Verification items for the finished model (mm, model axes). Face numbers are marked on the shaded views. A direction names the side the tool comes from. Coordinates: 2 decimals unless noted, no trailing zeros. Order: outer loops, then holes, each group sorted by start corner. A loop starts at its lowest first (then second) coordinate and runs counter-clockwise, first axis right, second up.
Q1. Cross-section at A-A, the plane z = 0. Record the boundary of the cut face in (x, y) (3 decimals), and give its area (3 significant figures).
Q2. Cross-section at D-D, the plane x = 0. Count the separate pieces of the cut face and the enclosed holes in it, and give its area (3 significant figures).
Q3. Cross-section at B-B, the plane y = 28.5. Record the boundary of the cut face in (x, z), and give its area (3 significant figures).
Q4. Set-up check for the marked faces 5, 6, 7, 8 and 9: record each of +Z, -Z, +X, -X, +Y, -Y from which the full face is reachable in a straight line by a thin tool's end or side.
Q5. Draft check along X on the marked faces 1, 2, 3 and 4. Enter one of: pulls with the +X half, pulls with the -X half, needs draft (parallel to the pull), parting line crosses it, or undercut.
Q6. Cross-section at C-C, the plane x = 34. Record the boundary of the cut face in (y, z) (3 decimals).
Q7. Depth check by flat-ended pin: P1, Ø5, axis at x = -36.5, y = 15.5, coming from the +Z side; P2, Ø12, axis at y = 26.5, z = -25.5, coming from the -X side; P3, Ø1, axis at x = -39, y = -20.5, coming from the +Z side. Enter the tip coordinate at first touch or a pass-through.
Q8. Thickness scan on line 1 (Z direction, x = 0, y = -4.8) (3 decimals); line 2 (Z direction, x = 0, y = 8); line 3 (Z direction, x = 0, y = 17.5). Record the ranges inside material, lowest first.
from build123d import *

# Parameters (mm, degrees)
F0_R      = 52.07
F1_DEPTH  = 5.08
F0_R_2    = 55.245
F2_DEPTH  = 30.48
F4_DEPTH  = 21.59
F5_W      = 9.2520020868
F5_H      = 19.05
F6_DEPTH  = 50.8
F7_W      = 9.2520020868
F7_H      = 19.05
F8_DEPTH  = 50.8
F9_W      = 9.2520020868
F9_H      = 19.05
F10_DEPTH = 50.8
F11_W     = 19.05
F11_H     = 9.2520020868
F12_DEPTH = 50.8
F13_W     = 19.05
F13_H     = 9.2520020868
F14_DEPTH = 50.8
F15_W     = 19.05
F15_H     = 9.2520020868
F16_DEPTH = 50.8
F17_W     = 9.2520020868
F17_H     = 19.05
F18_DEPTH = 50.8
F19_W     = 9.2520020868
F19_H     = 19.05
F20_DEPTH = 50.8
F21_W     = 9.2520020868
F21_H     = 19.05
F22_DEPTH = 50.8
F23_W     = 19.05
F23_H     = 9.2520020868
F24_DEPTH = 50.8
F25_W     = 19.05
F25_H     = 9.2520020868
F26_DEPTH = 50.8
F27_W     = 19.05
F27_H     = 9.2520020868
F28_DEPTH = 50.8
F29_W     = 40.64
F29_H     = 38.1
F30_DEPTH = 33.02
F31_DEPTH = 21.59
F33_DEPTH = 63.5
F34_W     = 20.2407714686
F34_H     = 6.3127256824
F35_DEPTH = 50.8
F36_W     = 16.5421865909
F36_H     = 6.3127256824
F37_DEPTH = 50.8
F38_W     = 20.32
F38_H     = 6.3127256824
F39_DEPTH = 50.8
F40_W     = 16.4780624607
F40_H     = 6.3127256824
F41_DEPTH = 50.8
F43_R     = 2.9464
F44_DEPTH = 1.6256
F42_R     = 11.811
F45_DEPTH = 36.83


with BuildPart() as f1:
    # F0 (on Front) → F1 (new body)
    with BuildSketch(Plane.XZ):
        Circle(F0_R)
    extrude(amount=F1_DEPTH)

    # F0 (on Front) → F2 (join)
    with BuildSketch(Plane.XZ):
        Circle(F0_R_2)
        Circle(F0_R, mode=Mode.SUBTRACT)
    extrude(amount=F2_DEPTH)

    # F3 (on face) → F4 (join)
    with BuildSketch(Plane.XZ.offset(5.08)):
        Polygon((4.5521322669, -17.2840948262), (12.5843095976, -12.6923990675), (17.2445313344, -4.6997852286), (17.2840948262, 4.5521322669), (12.6923990675, 12.5843095976), (4.6997852286, 17.2445313344), (-4.5521322669, 17.2840948262), (-12.5843095976, 12.6923990675), (-17.2445313344, 4.6997852286), (-17.2840948262, -4.5521322669), (-12.6923990675, -12.5843095976), (-4.6997852286, -17.2445313344), align=None)
    extrude(amount=F4_DEPTH)

    # F5 (on face) → F6 (cut)
    with BuildSketch(Plane(origin=(8.696092148, 0, 14.914420466), x_dir=(0.8638793813, 0, -0.5036987339), z_dir=(0.5036987339, 0, 0.8638793813))):
        with Locations((0, -17.145)):
            Rectangle(F5_W, F5_H)
    extrude(amount=F6_DEPTH, mode=Mode.SUBTRACT)

    # F7 (on face) → F8 (cut)
    with BuildSketch(Plane(origin=(0.0738264808, 0, 17.2643130803), x_dir=(0.999990857, 0, -0.0042762087), z_dir=(0.0042762087, 0, 0.999990857))):
        with Locations((0, -17.145)):
            Rectangle(F7_W, F7_H)
    extrude(amount=F8_DEPTH, mode=Mode.SUBTRACT)

    # F9 (on face) → F10 (cut)
    with BuildSketch(Plane(origin=(-8.5682209323, 0, 14.9882469469), x_dir=(0.86815559, 0, 0.4962921231), z_dir=(-0.4962921231, 0, 0.86815559))):
        with Locations((0, -17.145)):
            Rectangle(F9_W, F9_H)
    extrude(amount=F10_DEPTH, mode=Mode.SUBTRACT)

    # F11 (on face) → F12 (cut)
    with BuildSketch(Plane(origin=(-14.914420466, 0, 8.696092148), x_dir=(0, -1, 0), z_dir=(-0.8638793813, 0, 0.5036987339))):
        with Locations((17.145, 0)):
            Rectangle(F11_W, F11_H)
    extrude(amount=F12_DEPTH, mode=Mode.SUBTRACT)

    # F13 (on face) → F14 (cut)
    with BuildSketch(Plane(origin=(-17.2643130803, 0, 0.0738264808), x_dir=(0, -1, 0), z_dir=(-0.999990857, 0, 0.0042762087))):
        with Locations((17.145, 0)):
            Rectangle(F13_W, F13_H)
    extrude(amount=F14_DEPTH, mode=Mode.SUBTRACT)

    # F15 (on face) → F16 (cut)
    with BuildSketch(Plane(origin=(-14.9882469469, 0, -8.5682209323), x_dir=(0, -1, 0), z_dir=(-0.86815559, 0, -0.4962921231))):
        with Locations((17.145, 0)):
            Rectangle(F15_W, F15_H)
    extrude(amount=F16_DEPTH, mode=Mode.SUBTRACT)

    # F17 (on face) → F18 (cut)
    with BuildSketch(Plane(origin=(-8.696092148, 0, -14.914420466), x_dir=(0.8638793813, 0, -0.5036987339), z_dir=(-0.5036987339, 0, -0.8638793813))):
        with Locations((0, 17.145)):
            Rectangle(F17_W, F17_H)
    extrude(amount=F18_DEPTH, mode=Mode.SUBTRACT)

    # F19 (on face) → F20 (cut)
    with BuildSketch(Plane(origin=(-0.0738264808, 0, -17.2643130803), x_dir=(0.999990857, 0, -0.0042762087), z_dir=(-0.0042762087, 0, -0.999990857))):
        with Locations((0, 17.145)):
            Rectangle(F19_W, F19_H)
    extrude(amount=F20_DEPTH, mode=Mode.SUBTRACT)

    # F21 (on face) → F22 (cut)
    with BuildSketch(Plane(origin=(8.5682209323, 0, -14.9882469469), x_dir=(0.86815559, 0, 0.4962921231), z_dir=(0.4962921231, 0, -0.86815559))):
        with Locations((0, 17.145)):
            Rectangle(F21_W, F21_H)
    extrude(amount=F22_DEPTH, mode=Mode.SUBTRACT)

    # F23 (on face) → F24 (cut)
    with BuildSketch(Plane(origin=(14.914420466, 0, -8.696092148), x_dir=(0, 1, 0), z_dir=(0.8638793813, 0, -0.5036987339))):
        with Locations((-17.145, 0)):
            Rectangle(F23_W, F23_H)
    extrude(amount=F24_DEPTH, mode=Mode.SUBTRACT)

    # F25 (on face) → F26 (cut)
    with BuildSketch(Plane(origin=(17.2643130803, 0, -0.0738264808), x_dir=(0, 1, 0), z_dir=(0.999990857, 0, -0.0042762087))):
        with Locations((-17.145, 0)):
            Rectangle(F25_W, F25_H)
    extrude(amount=F26_DEPTH, mode=Mode.SUBTRACT)

    # F27 (on face) → F28 (cut)
    with BuildSketch(Plane(origin=(14.9882469469, 0, 8.5682209323), x_dir=(0, 1, 0), z_dir=(0.86815559, 0, 0.4962921231))):
        with Locations((-17.145, 0)):
            Rectangle(F27_W, F27_H)
    extrude(amount=F28_DEPTH, mode=Mode.SUBTRACT)

    # F29 (on face) → F30 (join)
    with BuildSketch(Plane.XZ):
        with Locations((0.0789208158, 0.021902828)):
            Rectangle(F29_W, F29_H)
    extrude(amount=-F30_DEPTH)

    # F31 (cut): a face of the model
    f31_faces = [f1.faces().sort_by_distance(p)[0] for p in [
        (0, -26.67, 0),
    ]]
    extrude(f31_faces, amount=-F31_DEPTH, mode=Mode.SUBTRACT)

    # F32 (on face) → F33 (join)
    with BuildSketch(Plane(origin=(0, 0, -19.028097172), x_dir=(1, 0, 0), z_dir=(0, 0, -1))):
        Polygon((-10.0810791842, -8.2228134091), (-10.0810791842, -24.765), (10.2389208158, -24.765), (10.2389208158, -8.2869375393), (10.1596922844, -8.2228134091), align=None)
    extrude(amount=F33_DEPTH)

    # F34 (on face) → F35 (join)
    with BuildSketch(Plane.XZ.offset(-8.2228134091)):
        with Locations((0.0393065501, -79.3717343307)):
            Rectangle(F34_W, F34_H)
    extrude(amount=F35_DEPTH)

    # F36 (on face) → F37 (join)
    with BuildSketch(Plane(origin=(-10.0810791842, 0, 0), x_dir=(0, -1, 0), z_dir=(-1, 0, 0))):
        with Locations((-16.4939067046, -79.3717343307)):
            Rectangle(F36_W, F36_H)
    extrude(amount=F37_DEPTH)

    # F38 (on face) → F39 (join)
    with BuildSketch(Plane(origin=(0, 24.765, 0), x_dir=(-1, 0, 0), z_dir=(0, 1, 0))):
        with Locations((-0.0789208158, -79.3717343307)):
            Rectangle(F38_W, F38_H)
    extrude(amount=F39_DEPTH)

    # F40 (on face) → F41 (join)
    with BuildSketch(Plane.YZ.offset(10.2389208158)):
        with Locations((16.5259687696, -79.3717343307)):
            Rectangle(F40_W, F40_H)
    extrude(amount=F41_DEPTH)

    # F43 (on face) → F44 (cut)
    with BuildSketch(Plane.XZ.offset(5.08)):
        Circle(F43_R)
    extrude(amount=-F44_DEPTH, mode=Mode.SUBTRACT)

    # F42 (on face) → F45 (cut)
    with BuildSketch(Plane(origin=(0, 33.02, 0), x_dir=(-1, 0, 0), z_dir=(0, 1, 0))):
        Circle(F42_R)
    extrude(amount=-F45_DEPTH, mode=Mode.SUBTRACT)


solid = f1.part
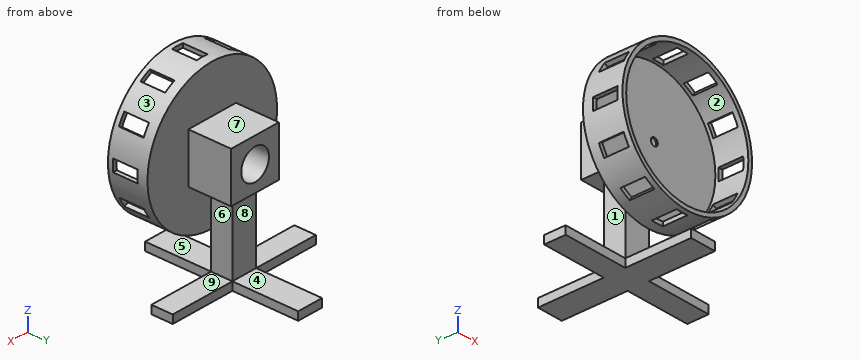
Check values:
1. outline: (-55.245, -30.48) - (-52.07, -30.48) - (-52.07, -26.67) - (-55.245, -26.67) - close; (-55.245, -7.62) - (-52.07, -7.62) - (-52.07, -5.08) - (-2.946, -5.08) - (-2.946, -3.81) - (-11.811, -3.81) - (-11.811, 33.02) - (-20.241, 33.02) - (-20.241, 0) - (-55.245, 0) - close; (2.946, -5.08) - (52.07, -5.08) - (52.07, -7.62) - (55.245, -7.62) - (55.245, 0) - (20.399, 0) - (20.399, 33.02) - (11.811, 33.02) - (11.811, -3.81) - (2.946, -3.81) - close; (52.07, -30.48) - (55.245, -30.48) - (55.245, -26.67) - (52.07, -26.67) - close
1. area: 1,070 mm2
2. separate pieces: 4
2. enclosed holes: 0
2. area: 2,670 mm2
3. outline: (-20.24, -19.03) - (20.4, -19.03) - (20.4, 19.07) - (-20.24, 19.07) - close; (-10.08, -82.53) - (10.24, -82.53) - (10.24, -76.22) - (-10.08, -76.22) - close; hole circle Ø23.62 at (0, 0)
3. area: 1,240 mm2
4. face 5: +X, -X, -Y
4. face 6: +X, +Y
4. face 7: +Z, +X, -X, +Y
4. face 8: +X, -X, +Y
4. face 9: +X, +Y, -Y
5. face 1: pulls with the -X half
5. face 2: undercut
5. face 3: parting line crosses it
5. face 4: needs draft
6. outline: (-30.48, -43.543) - (0, -43.543) - (0, 43.543) - (-30.48, 43.543) - (-30.48, 39.437) - (-5.08, 39.437) - (-5.08, -39.437) - (-30.48, -39.437) - close; (8.287, -82.528) - (24.765, -82.528) - (24.765, -76.215) - (8.287, -76.215) - close
7. P1: stops at z = -76.22
7. P2: stops at x = -10.08
7. P3: stops at z = 39.62
8. line 1: z = -82.528 to -76.215, -55.245 to -2.946, 2.946 to 55.245
8. line 2: z = -82.53 to -76.22, -19.03 to -11.81, 11.81 to 19.07
8. line 3: z = -82.53 to -11.81, 11.81 to 19.07
